Geometry check sheet. Reference: the model listing, model coordinates, mm. Face numbers are marked on the shaded views. Round coordinates to 2 decimals unless told otherwise and drop trailing zeros. Order: outer loops, then holes, each group sorted by start corner. A loop starts at its lowest first (then second) coordinate and runs counter-clockwise, first axis right, second up. Notation, with made-up numbers: (56, 0.5) - (88, 0.5) arc R34 ccw to (88, 32.5) - close; hole circle Ø4 at (71, 88). An arc over 180 degrees is marked (long way). Use a Markdown table: item, result. Add a question column.
(1) Section check D-D on z = 4.75. Record the boundary of the cut face in (x, y) (1 decimal), then the cut area to 3 significant figures.
(2) Section check C-C on x = 4.5. Record the boundary of the cut face in (y, z), then the cut area to 3 significant figures.
(3) Mould release check, pull along Y, two halves, no side actions. Record for the marked faces 1, 2 and 3: released by +Y, released by -Y, zero draft, split by the parting line, or undercut.
(4) Section check B-B on y = 35. Record the boundary of the cut face in (x, z).
(5) Gauge pin test, flat ends, axial feed: P1, Ø2, axis at y = -64, z = 8, coming from the +X side; P2, Ø6, axis at y = 38, z = 3.5, coming from the +X side; P3, Ø3, axis at y = -29.5, z = 4.5, coming from the +X side. Record the tip position at first contact, or that the pin passes through.
(6) Section check A-A on x = -35. Record the boundary of the cut face in (y, z), then the cut area to 3 significant figures.
(7) Thickness scan on line 1 along Y through (x, z) = (0, 5.25); line 2 along Y through (x, z) = (35, 5.5); line 3 along X through (y, z) = (32.5, 9). Record the ranges inside material, lowest first. Write a range as [from, to].
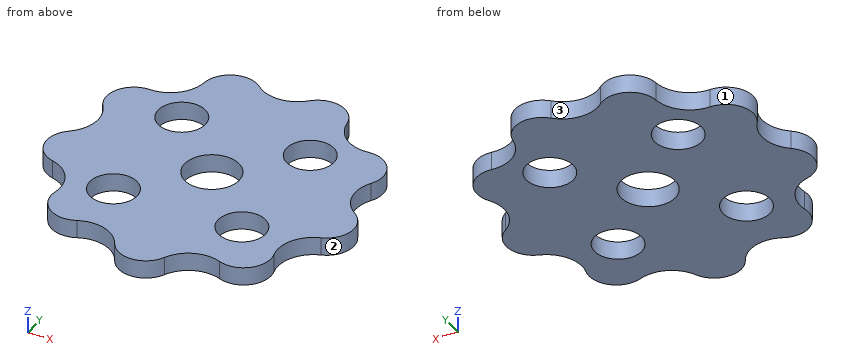
```python
from build123d import *

# Parameters (mm, degrees)
BOSS_EXTRUDE1_DEPTH = 10
SKETCH3_R           = 13
SKETCH3_R_2         = 15
CUT_EXTRUDE1_DEPTH  = 120.101165428


with BuildPart() as part:
    # Sketch1 → Boss-Extrude1 (new body)
    with BuildSketch(Plane.XY):
        with BuildLine():
            ThreePointArc((-14.43044528, 75.890215107), (-0.949427503, 70.727267405), (12.388145038, 76.250222049))
            ThreePointArc((12.388145038, 76.250222049), (27.789798404, 79.662981363), (37.726927549, 67.410988998))
            ThreePointArc((37.726927549, 67.410988998), (44.735307492, 54.790510408), (58.502567636, 50.44811275))
            ThreePointArc((58.502567636, 50.44811275), (72.494598013, 43.162446106), (72.23145169, 27.389411947))
            ThreePointArc((72.23145169, 27.389411947), (69.487894935, 13.216664662), (77.242988653, 1.040770827))
            ThreePointArc((77.242988653, 1.040770827), (83.278369525, -13.534277382), (72.938076822, -25.447975353))
            ThreePointArc((72.938076822, -25.447975353), (61.726324065, -34.541405366), (59.84055682, -48.853559333))
            ThreePointArc((59.84055682, -48.853559333), (55.0952664, -63.898162065), (39.516165192, -66.377972163))
            ThreePointArc((39.516165192, -66.377972163), (25.082320154, -66.137167939), (14.438063397, -75.888766134))
            ThreePointArc((14.438063397, -75.888766134), (1.13247581, -84.36338657), (-12.395799304, -76.248978089))
            ThreePointArc((-12.395799304, -76.248978089), (-23.297980116, -66.7866146), (-37.720160351, -67.414775851))
            ThreePointArc((-37.720160351, -67.414775851), (-53.360212797, -65.354044903), (-58.507631542, -50.442239754))
            ThreePointArc((-58.507631542, -50.442239754), (-60.776896562, -36.185862039), (-72.228701857, -27.396662716))
            ThreePointArc((-72.228701857, -27.396662716), (-82.885064803, -15.764819298), (-77.243092741, -1.033016835))
            ThreePointArc((-77.243092741, -1.033016835), (-69.817627646, 11.34665753), (-72.940631032, 25.440653384))
            ThreePointArc((-72.940631032, 25.440653384), (-73.627073824, 41.200940464), (-59.835652386, 48.859566142))
            ThreePointArc((-59.835652386, 48.859566142), (-46.189914818, 53.569949938), (-39.522828302, 66.374005024))
            ThreePointArc((-39.522828302, 66.374005024), (-29.918156728, 78.888322285), (-14.43044528, 75.890215107))
        make_face()
    extrude(amount=BOSS_EXTRUDE1_DEPTH)

    # Sketch3 → Cut-Extrude1 (cut, through all)
    with BuildSketch(Plane(origin=(0, 0, 0), x_dir=(-1, 0, 0), z_dir=(0, 0, -1))):
        with Locations((-35, 35)):
            Circle(SKETCH3_R)
        with Locations((35, 35)):
            Circle(SKETCH3_R)
        with Locations((35, -35)):
            Circle(SKETCH3_R)
        with Locations((-35, -35)):
            Circle(SKETCH3_R)
        Circle(SKETCH3_R_2)
    extrude(amount=-CUT_EXTRUDE1_DEPTH, mode=Mode.SUBTRACT)


solid = part.part
```
Check sheet entries:
| question | item | result |
|---|---|---|
| 1 | outline | (-77.2, -1) arc R15 ccw to (-72.2, -27.4) arc R19.5 cw to (-58.5, -50.4) arc R15 ccw to (-37.7, -67.4) arc R19.5 cw to (-12.4, -76.2) arc R15 ccw to (14.4, -75.9) arc R19.5 cw to (39.5, -66.4) arc R15 ccw to (59.8, -48.9) arc R19.5 cw to (72.9, -25.4) arc R15 ccw to (77.2, 1) arc R19.5 cw to (72.2, 27.4) arc R15 ccw to (58.5, 50.4) arc R19.5 cw to (37.7, 67.4) arc R15 ccw to (12.4, 76.3) arc R19.5 cw to (-14.4, 75.9) arc R15 ccw to (-39.5, 66.4) arc R19.5 cw to (-59.8, 48.9) arc R15 ccw to (-72.9, 25.4) arc R19.5 cw to start; hole circle Ø26 at (-35, -35); hole circle Ø26 at (-35, 35); hole circle Ø30 at (0, 0); hole circle Ø26 at (35, -35); hole circle Ø26 at (35, 35) |
| 1 | area | 16,100 mm2 |
| 2 | outline | (-83.93, 0) - (-14.31, 0) - (-14.31, 10) - (-83.93, 10) - close; (14.31, 0) - (71.58, 0) - (71.58, 10) - (14.31, 10) - close |
| 2 | area | 1,270 mm2 |
| 3 | face 1 | undercut |
| 3 | face 2 | split by the parting line |
| 3 | face 3 | released by +Y |
| 4 | outline | (-75.5, 0) - (-48, 0) - (-48, 10) - (-75.5, 10) - close; (-22, 0) - (22, 0) - (22, 10) - (-22, 10) - close; (48, 0) - (74.6, 0) - (74.6, 10) - (48, 10) - close |
| 5 | P1 | stops at x = 56.05 |
| 5 | P2 | stops at x = 74.61 |
| 5 | P3 | stops at x = 67.69 |
| 6 | outline | (-66.43, 0) - (-48, 0) - (-48, 10) - (-66.43, 10) - close; (-22, 0) - (22, 0) - (22, 10) - (-22, 10) - close; (48, 0) - (75.67, 0) - (75.67, 10) - (48, 10) - close |
| 6 | area | 901 mm2 |
| 7 | line 1 | y = [-84.34, -15], [15, 70.76] |
| 7 | line 2 | y = [-65.1, -48], [-22, 22], [48, 74.3] |
| 7 | line 3 | x = [-75.47, -47.76], [-22.24, 22.24], [47.76, 74.31] |
